For this review, take the finished solid that the model builds, in its own axes (mm). A direction names the side the tool comes from. Round coordinates to 2 decimals unless told otherwise and drop trailing zeros. Write each loop counter-clockwise with the first axis right and the second up, starting at its lowest first coordinate (ties: lowest second). Pieces come first, ordered by that corner, then holes. Notation, with made-up numbers: (85.25, 33) -> (133.25, 33) arc R25 ccw to (133.25, 46) -> close; hole circle Ø1 at (23, -34). An arc over 180 degrees is marked (long way). Answer in a Markdown table with one row per item.
from build123d import *

# Parameters (mm, degrees)
SALIENTE_EXTRUIR1_DEPTH = 1
CROQUIS2_W              = 64
CROQUIS2_H              = 60
SALIENTE_EXTRUIR2_DEPTH = 50


with BuildPart() as part:
    # Croquis1 → Saliente-Extruir1 (new body)
    with BuildSketch(Plane(origin=(0, 0, 0), x_dir=(1, 0, 0), z_dir=(0, 1, 0))):
        Polygon((-32, 11.5), (-45, 11.5), (-45, -11.5), (-32, -11.5), (-32, -30), (32, -30), (32, -11.5), (45, -11.5), (45, 11.5), (32, 11.5), (32, 30), (-32, 30), align=None)
        with BuildLine():
            Line((-40.5, -2.5), (-36.5, -2.5))
            ThreePointArc((-36.5, -2.5), (-34, 0), (-36.5, 2.5))
            Line((-36.5, 2.5), (-40.5, 2.5))
            ThreePointArc((-40.5, 2.5), (-43, 0), (-40.5, -2.5))
        make_face(mode=Mode.SUBTRACT)
        with BuildLine():
            Line((40.5, -2.5), (36.5, -2.5))
            ThreePointArc((36.5, -2.5), (34, 0), (36.5, 2.5))
            Line((36.5, 2.5), (40.5, 2.5))
            ThreePointArc((40.5, 2.5), (43, 0), (40.5, -2.5))
        make_face(mode=Mode.SUBTRACT)
    extrude(amount=SALIENTE_EXTRUIR1_DEPTH)

    # Croquis2 → Saliente-Extruir2 (add)
    with BuildSketch(Plane(origin=(0, 1, 0), x_dir=(1, 0, 0), z_dir=(0, 1, 0))):
        Rectangle(CROQUIS2_W, CROQUIS2_H)
    extrude(amount=SALIENTE_EXTRUIR2_DEPTH)


solid = part.part
1) Consider section C-C on z = 8. State the section outline as (x, y) points.
Solved:
| item | result |
|---|---|
| outline | (-45, 0) -> (45, 0) -> (45, 1) -> (32, 1) -> (32, 51) -> (-32, 51) -> (-32, 1) -> (-45, 1) -> close |
2) Mouldability with a two-part tool opening along X and no side actions: class faces 1 (the flat face through (-1, 0, 0)), 2 (the cylindrical face through (34, 0.5, 0.1)) as pulls with the +X half, pulls with the -X half, needs draft (parallel to the pull), parting line crosses it, or undercut.
Solved:
| item | result |
|---|---|
| face 1 | needs draft |
| face 2 | undercut |
3) Consider section B-B on x = 35. State the section outline as (y, z) points.
Solved:
| item | result |
|---|---|
| outline | (0, -11.5) -> (1, -11.5) -> (1, -2) -> (0, -2) -> close; (0, 2) -> (1, 2) -> (1, 11.5) -> (0, 11.5) -> close |
4) For line 1 (X direction, y = 44, z = -2); line 2 (Y direction, x = -32.5, z = 7.5), list the stretches that pass through material, from the lowest coordinate up. Write a range as [from, to].
Solved:
| item | result |
|---|---|
| line 1 | [-32, 32] |
| line 2 | [0, 1] |
5) For faces 3 (the cylindrical face through (43, 0.5, -0.1)), 4 (the flat face through (38, 1, -3)), 5 (the flat face through (-39, 1, -3)), list the 3-axis set-ups (+Z, -Z, +X, -X, +Y, -Y) from which the entire face can be reached by the end or side of a thin tool; tool diameter is ignored.
Solved:
| item | result |
|---|---|
| face 3 | +Y, -Y |
| face 4 | +Z, -Z, +X, +Y |
| face 5 | +Z, -Z, -X, +Y |
6) Consider section D-D on y = 42. State the section outline as (x, z) points, then the cut area to 3 significant figures.
Solved:
| item | result |
|---|---|
| outline | (-32, -30) -> (32, -30) -> (32, 30) -> (-32, 30) -> close |
| area | 3,840 mm² |
7) Clearance check with flat-ended pins moving along their axes: pin 1 Ø12 at (y, z) = (37, -4.5) entering from -X; pin 2 Ø14.5 at (x, z) = (39.5, 1.5) entering from +Y; pin 3 Ø0.5 at (x, y) = (38, 0.5) entering from +Z; pin 4 Ø8 at (x, z) = (25, -6.5) entering from -Y. State where each tip first meets the part, or that it passes through.
Solved:
| item | result |
|---|---|
| pin 1 | x = -32 |
| pin 2 | y = 1 |
| pin 3 | z = 11.5 |
| pin 4 | y = 0 |
8) Consider section A-A on z = 0. State the section outline as (x, y) points.
Solved:
| item | result |
|---|---|
| outline | (-45, 0) -> (-43, 0) -> (-43, 1) -> (-45, 1) -> close; (-34, 0) -> (34, 0) -> (34, 1) -> (32, 1) -> (32, 51) -> (-32, 51) -> (-32, 1) -> (-34, 1) -> close; (43, 0) -> (45, 0) -> (45, 1) -> (43, 1) -> close |
